```python
from build123d import *

# Parameters (mm, degrees)
SKETCH5_W                                    = 29
SKETCH5_H                                    = 37
BOSS_EXTRUDE3_DEPTH                          = 0.5
SKETCH6_R                                    = 1.095
CUT_EXTRUDE1_DEPTH                           = 1
CUT_EXTRUDE1_DEPTH_BACK                      = 1.5
SKETCH7_W                                    = 29
SKETCH7_H                                    = 37
BOSS_EXTRUDE4_DEPTH                          = 1
FILLET1_R                                    = 3
CSK_FOR_M3_COUNTERSUNK_FLAT_HEAD_SCR_2_COUNT = 2
CSK_FOR_M3_COUNTERSUNK_FLAT_HEAD_SCR_2_PITCH = 22
CSK_FOR_M3_COUNTERSUNK_FLAT_HEAD_SCR_3_COUNT = 2
CSK_FOR_M3_COUNTERSUNK_FLAT_HEAD_SCR_3_PITCH = 37.202150475
CSK_FOR_M3_COUNTERSUNK_FLAT_HEAD_SCR_4_COUNT = 2
CSK_FOR_M3_COUNTERSUNK_FLAT_HEAD_SCR_4_PITCH = 30


with BuildPart() as part:
    # Sketch5 → Boss-Extrude3 (new body)
    with BuildSketch(Plane(origin=(0, 0, 0), x_dir=(1, 0, 0), z_dir=(0, 1, 0))):
        Rectangle(SKETCH5_W, SKETCH5_H)
    extrude(amount=BOSS_EXTRUDE3_DEPTH)

    # Sketch6 → Cut-Extrude1 (cut, two sides)
    with BuildSketch(Plane(origin=(0, 0.5, 0), x_dir=(1, 0, 0), z_dir=(0, 1, 0))) as cut_extrude1_sk:
        with Locations((-6.025, 0)):
            Circle(SKETCH6_R)
        with Locations((6.025, 0)):
            Circle(SKETCH6_R)
    extrude(amount=CUT_EXTRUDE1_DEPTH, mode=Mode.SUBTRACT)
    extrude(cut_extrude1_sk.sketch, amount=-CUT_EXTRUDE1_DEPTH_BACK, mode=Mode.SUBTRACT)

    # Sketch7 → Boss-Extrude4 (add)
    with BuildSketch(Plane(origin=(0, 0.5, 0), x_dir=(1, 0, 0), z_dir=(0, 1, 0))):
        Rectangle(SKETCH7_W, SKETCH7_H)
        with BuildLine():
            ThreePointArc((4.362935735, -8.496468579), (6.43071599, -7.092318659), (8.065752838, -5.201814312))
            Line((8.065752838, -5.201814312), (8.065752838, 5.280856896))
            ThreePointArc((8.065752838, 5.280856896), (0.065752838, 9.758587375), (-7.934247162, 5.280856896))
            Line((-7.934247162, 5.280856896), (-7.934247162, -5.211512098))
            ThreePointArc((-7.934247162, -5.211512098), (-6.328814647, -7.036583971), (-4.385354374, -8.496468579))
            Line((-4.385354374, -8.496468579), (4.362935735, -8.496468579))
        make_face(mode=Mode.SUBTRACT)
    extrude(amount=BOSS_EXTRUDE4_DEPTH)

    # Fillet1
    fillet1_edges = [part.edges().sort_by_distance(p)[0] for p in [
        (-14.5, 0.75, -18.5),
        (14.5, 0.75, -18.5),
        (14.5, 0.75, 18.5),
        (-14.5, 0.75, 18.5),
    ]]
    fillet(fillet1_edges, radius=FILLET1_R)

    # Sketch11 → CSK for M3 Countersunk Flat Head Screw1 (revolve, cut)
    with BuildSketch(Plane(origin=(-11, 0, -15), x_dir=(0, 0, -1), z_dir=(1, 0, 0))):
        Polygon((0, 0), (0, 1.5), (1.7, 1.5), (1.7, 1.45), (3.15, 0), align=None)
    csk_for_m3_countersunk_flat_head_screw1 = revolve(axis=Axis((-11, -6.35, -15), (0, 1, 0)), mode=Mode.SUBTRACT)

    # CSK for M3 Countersunk Flat Head Scr 2: CSK for M3 Countersunk Flat Head Screw1 ×2
    with Locations(*[(i * CSK_FOR_M3_COUNTERSUNK_FLAT_HEAD_SCR_2_PITCH, 0, 0) for i in range(1, CSK_FOR_M3_COUNTERSUNK_FLAT_HEAD_SCR_2_COUNT)]):
        add(csk_for_m3_countersunk_flat_head_screw1, mode=Mode.SUBTRACT)

    # CSK for M3 Countersunk Flat Head Scr 3: CSK for M3 Countersunk Flat Head Screw1 ×2
    with Locations(*[Vector(0.591363664, 0, 0.806404996) * (i * CSK_FOR_M3_COUNTERSUNK_FLAT_HEAD_SCR_3_PITCH) for i in range(1, CSK_FOR_M3_COUNTERSUNK_FLAT_HEAD_SCR_3_COUNT)]):
        add(csk_for_m3_countersunk_flat_head_screw1, mode=Mode.SUBTRACT)

    # CSK for M3 Countersunk Flat Head Scr 4: CSK for M3 Countersunk Flat Head Screw1 ×2
    with Locations(*[(0, 0, i * CSK_FOR_M3_COUNTERSUNK_FLAT_HEAD_SCR_4_PITCH) for i in range(1, CSK_FOR_M3_COUNTERSUNK_FLAT_HEAD_SCR_4_COUNT)]):
        add(csk_for_m3_countersunk_flat_head_screw1, mode=Mode.SUBTRACT)


solid = part.part
```
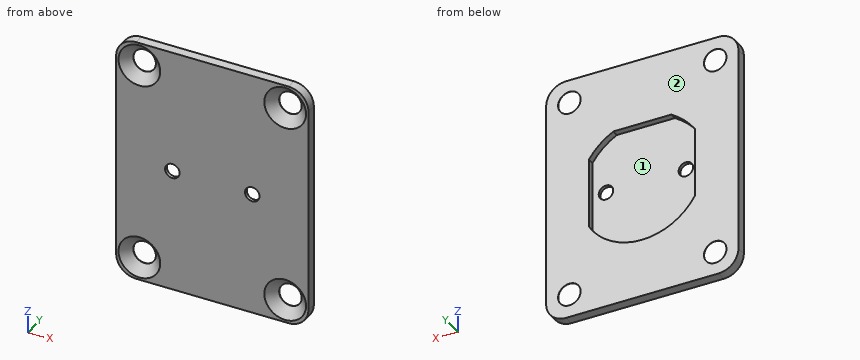
Could you check a few things on this model? Use its own coordinates, in mm. Face numbers are marked on the shaded views. A direction names the side the tool comes from. Coordinates: 2 decimals unless noted, no trailing zeros. Order: outer loops, then holes, each group sorted by start corner. A loop starts at its lowest first (then second) coordinate and runs counter-clockwise, first axis right, second up. Notation, with made-up numbers: M 44,44.5 L 95,44.5 A17 cw 95,73.5 Z; hole C 51,-25 d5. An arc over 180 degrees is marked long. Use a Markdown table: item, result. Add a question column.
Q1. I want a section at A-A on x = 11. List the corners of the cut face in (y, z) for me, then the cut area to 3 significant figures.
Q2. I want a section at C-C on x = -6.5. List the corners of the cut face in (y, z) for me.
Q3. Which directions (+Z, -Z, +X, -X, +Y, -Y) give clear straight access to the entire face, cutting with the end or side of a thin tool? Please do the marked faces 1 and 2.
Q4. I want a section at B-B on z = 15. List the corners of the cut face in (x, y) for me.
Q5. If I drill on L1, parallel to X at y = 0.25, z = 0; L2, parallel to X at y = 0.75, z = 16.5; L3, parallel to Z at x = 0.5, y = 0.7, over which ranges is the centre line in solid material (lowest first)?
Q6. I want a section at D-D on z = 4.5. List the corners of the cut face in (x, y) for me.
Q7. I'm going to push flat-ended pins straight in: pin 1 (2.5 mm diameter, centred on x = 11, z = 15, fed in from +Y); pin 2 (3 mm diameter, centred on x = -6.025, z = 0, fed in from -Y); pin 3 (8 mm diameter, centred on x = 3.5, z = 3.5, fed in from +Y). Where does each tip first touch, or does it pass through?
Checked values:
| question | item | result |
|---|---|---|
| 1 | outline | M 0,-18.5 L 1.5,-18.5 L 1.5,-16.7 L 1.45,-16.7 L 0,-18.15 Z; M 0,-11.85 L 1.45,-13.3 L 1.5,-13.3 L 1.5,13.3 L 1.45,13.3 L 0,11.85 Z; M 0,18.15 L 1.45,16.7 L 1.5,16.7 L 1.5,18.5 L 0,18.5 Z |
| 1 | area | 41.1 mm² |
| 2 | outline | M 0,-18.5 L 1.5,-18.5 L 1.5,-7.08 L 0.5,-7.08 L 0.5,-0.99 L 0,-0.99 Z; M 0,0.99 L 0.5,0.99 L 0.5,6.87 L 1.5,6.87 L 1.5,18.5 L 0,18.5 Z |
| 3 | face 1 | +Y |
| 3 | face 2 | +Z, -Z, +X, -X, +Y |
| 4 | outline | M -14.5,0 L -14.15,0 L -12.7,1.45 L -12.7,1.5 L -14.5,1.5 Z; M -9.3,1.45 L -7.85,0 L 7.85,0 L 9.3,1.45 L 9.3,1.5 L -9.3,1.5 Z; M 12.7,1.45 L 14.15,0 L 14.5,0 L 14.5,1.5 L 12.7,1.5 Z |
| 5 | L1 | -14.5 to -7.12, -4.93 to 4.93, 7.12 to 14.5 |
| 5 | L2 | -14.33 to -12.87, -9.13 to 9.13, 12.87 to 14.33 |
| 5 | L3 | -18.5 to -9.75, 8.5 to 18.5 |
| 6 | outline | M -14.5,0 L 14.5,0 L 14.5,1.5 L 8.07,1.5 L 8.07,0.5 L -7.93,0.5 L -7.93,1.5 L -14.5,1.5 Z |
| 7 | pin 1 | through |
| 7 | pin 2 | y = 0 |
| 7 | pin 3 | y = 0.5 |
